Autodesk Inventor part; units mm, degrees
ref_plane "YZ Plane" through (0, 0, 0) normal (1, 0, 0) x (0, 1, 0)
ref_plane "XZ Plane" through (0, 0, 0) normal (0, 1, 0) x (-1, 0, 0)
ref_plane "XY Plane" through (0, 0, 0) normal (0, 0, 1) x (1, 0, 0)
sketch "Sketch2" plane through (0, 0, 0) normal (1, 0, 0) x (0, 1, 0)
  line L0 (-29.4, 0) -> (29.4, 0) construction
  line L1 (0, -71.4) -> (0, 71.4) construction
  line L2 (1.5, -46) -> (1.5, -48)
  line L3 (-1.5, -46) -> (-1.5, -48)
  line L4 (1.5, -46) -> (2.65, -46)
  line L5 (2.65, -43.6) -> (2.65, -46)
  line L6 (2.65, -43.6) -> (1.5, -43.6)
  line L7 (1.5, -43.6) -> (1.5, -43)
  line L8 (1.5, -43) -> (-1.5, -43)
  line L9 (-1.5, -43) -> (-1.5, -43.6)
  line L10 (-2.65, -43.6) -> (-1.5, -43.6)
  line L11 (-2.65, -43.6) -> (-2.65, -46)
  line L12 (-1.5, -46) -> (-2.65, -46)
  line L13 (1.5, -48) -> (9, -48)
  line L14 (9, -51) -> (9, -48)
  line L15 (-1.5, -48) -> (-9, -48)
  line L16 (3.975, -48) -> (3.975, -51)
  line L17 (9, -51) -> (3.975, -51)
  line L18 (-9, -48) -> (-9, -51)
  line L19 (-9, -51) -> (-3.975, -51)
  line L20 (-3.975, -51) -> (-3.975, -48)
  line L21 (9, -48) -> (10.5, -48)
  line L22 (-9, -48) -> (-10.5, -48)
  line L23 (2.65, 43.6) -> (2.65, 46)
  line L24 (2.65, 46) -> (-2.65, 46)
  line L25 (-2.65, 46) -> (-2.65, 43.6)
  line L26 (-2.65, 43.6) -> (2.65, 43.6)
  line L27 (-10.5, 48) -> (-9, 48)
  line L28 (1.5, 46) -> (1.5, 48)
  line L29 (-1.5, 46) -> (-1.5, 48)
  line L30 (1.5, 43.6) -> (1.5, 43)
  line L31 (1.5, 43) -> (-1.5, 43)
  line L32 (-1.5, 43) -> (-1.5, 43.6)
  line L33 (9, 51) -> (9, 48)
  line L34 (3.975, 48) -> (3.975, 51)
  line L35 (9, 51) -> (3.975, 51)
  line L36 (-9, 48) -> (-9, 51)
  line L37 (-9, 51) -> (-3.975, 51)
  line L38 (-3.975, 51) -> (-3.975, 48)
  line L39 (9, 48) -> (21, 48)
  line L40 (-9, 48) -> (-10.5, 48)
  line L41 (21, 48) -> (21, -48)
  line L42 (-21, -48) -> (-21, 48)
  line L43 (3.975, 48) -> (9, 48)
  line L44 (-3.975, 48) -> (3.975, 48)
  line L45 (-9, 48) -> (-3.975, 48)
  line L46 (10.5, -48) -> (21, -48)
  line L47 (-10.5, -48) -> (-21, -48)
  line L48 (-10.5, 48) -> (-21, 48)
  line L49 (9, 48) -> (10.5, 48)
  circle A0 centre (0, 0) radius 11.5
  circle A1 centre (0, 30.8333) radius 3.9
  circle A2 centre (0, -30.8333) radius 3.9
  line L50 (2.65, 46) -> (2.65, 43.6)
  line L51 (2.65, 43.6) -> (-2.65, 43.6)
  line L52 (-2.65, 43.6) -> (-2.65, 46)
  line L53 (-2.65, 46) -> (2.65, 46)
  line L54 (2.65, -43.6) -> (2.65, -46)
  line L55 (2.65, -46) -> (-2.65, -46)
  line L56 (-2.65, -46) -> (-2.65, -43.6)
  line L57 (-2.65, -43.6) -> (2.65, -43.6)
  circle A3 centre (15.5, -15.5) radius 1.4
  circle A4 centre (-15.5, -15.5) radius 1.4
  circle A5 centre (-15.5, 15.5) radius 1.4
  circle A6 centre (15.5, 15.5) radius 1.4
  line L58 (-21, -51) -> (-10.5, -51)
  line L59 (-10.5, -51) -> (-10.5, -48)
  line L60 (-10.5, -48) -> (10.5, -48)
  line L61 (10.5, -48) -> (10.5, -51)
  line L62 (10.5, -51) -> (21, -51)
  line L63 (21, -51) -> (21, 51)
  line L64 (21, 51) -> (10.5, 51)
  line L65 (10.5, 51) -> (10.5, 48)
  line L66 (10.5, 48) -> (-10.5, 48)
  line L67 (-10.5, 48) -> (-10.5, 51)
  line L68 (-10.5, 51) -> (-21, 51)
  line L69 (-21, 51) -> (-21, -51)
  dimension "d4" = 3
  dimension "d6" = 7.95
  dimension "d8" = 5
extrude "Extrusion1" add sketch "Sketch2" along normal blind 3 contours L4 L5 L6 L7 L8 L9 L10 L11 L12 L3 L15 L22 L47 L42 L48 L27 L45 L44 L29 L24 L25 L26 L32 L31 L30 L23 L28 L43 L39 L41 L46 L21 L13 L2 | L13 L14 L17 L16 | L20 L19 L18 L15 | L43 L34 L35 L33 | L36 L37 L38 L45
properties part number "Front-Outer"
Model file for the job. Use its own axes, mm. A direction names the side the tool comes from. Round coordinates to 2 decimals unless told otherwise and drop trailing zeros. Loops run counter-clockwise (first coordinate to the right, second up) from the corner with the lowest first, then second, coordinate; pieces in that order, holes last.
1. Tool access for faces 4 (the flat face through (1, 9, 50)), 5 (the flat face through (1, -15, 48)), 6 (the flat face through (1, 0, 43)): list every direction of +Z, -Z, +X, -X, +Y, -Y with a clear straight run to the whole face (end or side of a thin tool).
Check values:
face 4: +Z, +X, -X, +Y
face 5: +Z, +X, -X, -Y
face 6: +Z, +X, -X
2. Band-saw the part on A-A, the plane z = 0. List the corners of the cut face in (x, y), and give its area (3 significant figures).
Check values:
outline: (0, -21) - (3, -21) - (3, -11.5) - (0, -11.5) - close; (0, 11.5) - (3, 11.5) - (3, 21) - (0, 21) - close
area: 57.0 mm2
3. Wall check: probe 1 along Z at (x, y) = (1.05, 15.5); probe 2 along Z at (x, y) = (1.9, 0); probe 3 along Y at (x, z) = (2, 30.5). Give the ranges that are in metal, low to high.
Check values:
probe 1: z = -48 to -16.9, -14.1 to 14.1, 16.9 to 48
probe 2: z = -43 to -34.73, -26.93 to -11.5, 11.5 to 26.93, 34.73 to 43
probe 3: y = -21 to -3.89, 3.89 to 21
4. Band-saw the part on D-D, the plane y = -15. List the corners of the cut face in (x, z), and give its area (3 significant figures).
Check values:
outline: (0, -48) - (3, -48) - (3, -16.81) - (0, -16.81) - close; (0, -14.19) - (3, -14.19) - (3, 14.19) - (0, 14.19) - close; (0, 16.81) - (3, 16.81) - (3, 48) - (0, 48) - close
area: 272 mm2
5. Band-saw the part on C-C, the plane z = 15.5. List the corners of the cut face in (x, y).
Check values:
outline: (0, -21) - (3, -21) - (3, -16.9) - (0, -16.9) - close; (0, -14.1) - (3, -14.1) - (3, 14.1) - (0, 14.1) - close; (0, 16.9) - (3, 16.9) - (3, 21) - (0, 21) - close
6. Mould opens along Z. For faces 1 (the flat face through (1, -2.65, 45)), 2 (the flat face through (3, 0, 12)), 3 (the flat face through (1, -7, 51)) say: +Z half, -Z half, draft (parallel to the pull), parting line (faces both ways), or undercut.
Check values:
face 1: undercut
face 2: draft
face 3: +Z half
7. Drop flat-ended pins along their axis: P1, Ø1.5, axis at x = 2, y = 15.5, coming from the +Z side; P2, Ø0.9, axis at x = 1, z = 49.5, coming from the -Y side. Give the stop position or say it passes through.
Check values:
P1: stops at z = 48
P2: stops at y = -9
8. Band-saw the part on B-B, the plane y = 0. List the corners of the cut face in (x, z).
Check values:
outline: (0, -43) - (3, -43) - (3, -34.73) - (0, -34.73) - close; (0, -26.93) - (3, -26.93) - (3, -11.5) - (0, -11.5) - close; (0, 11.5) - (3, 11.5) - (3, 26.93) - (0, 26.93) - close; (0, 34.73) - (3, 34.73) - (3, 43) - (0, 43) - close
